Can you work these out from the model? Positions are in its coordinate system, mm. A direction names the side the tool comes from. Coordinates: 2 decimals unless noted, no trailing zeros. Loops run counter-clockwise (first coordinate to the right, second up) from the corner with the lowest first, then second, coordinate; pieces in that order, holes last. Notation, with made-up numbers: (35.5, 18.25) -> (44.5, 18.25) arc R16 ccw to (44.5, 48.25) -> close; hole circle Ø4 at (34, 53). An arc over 180 degrees is marked (long way). Put each result on its own line as item: value. Start each with the question number.
Item 1: If we section it at B-B on y = 0: Please give me the cut outline in (x, z), plus the area to 3 significant figures.
Item 2: For faces 1 (the cylindrical face through (-32.1, -32.14, -5.93)), 2 (the cylindrical face through (41, 41.07, -7.34)), 3 (the flat face through (0, 39.4, -7)), 4 (the cylindrical face through (0.404, -40.972, -10.074)), which set-ups out of +Z, -Z, +X, -X, +Y, -Y let a thin tool reach every point of the face, with its end or its side?
Item 3: If we section it at D-D on y = 24: Please give me the cut outline in (x, z).
Item 4: Will these pins go through, and if not, where does the flat tip stop? P1, Ø6.5, axis at x = -3, y = -28, coming from the +Z side; P2, Ø5.5, axis at y = 0, z = -7, coming from the -X side; P3, Ø1, axis at x = 16, y = 20, coming from the +Z side.
Item 5: We'd pull the mould along Z, two halves only. Please class faces 5 (the flat face through (-39.4, 0, -7)), 6 (the cylindrical face through (0.52, -41.07, -17)), 7 (the flat face through (-18, 33, -6)): pulls with the +Z half, pulls with the -Z half, needs draft (parallel to the pull), parting line crosses it, or undercut.
Item 6: If we section it at A-A on x = 0: Please give me the cut outline in (y, z).
Item 7: Please list where these lines run through material, in increasing order: L1, parallel to Y at x = 16, z = -9; L2, parallel to X at y = -8.5, z = -7; L3, parallel to X at y = 30.5, z = -10. Write a range as from..to.
Item 8: If we section it at C-C on z = -7: State how many separate pieces and enclosed holes the cut face has, plus the area to 3 significant figures.
```python
from build123d import *

# Parameters (mm, degrees)
F0_W      = 85
F0_H      = 85
F0_R      = 2
F3_DEPTH  = 18.5
F4_DEPTH  = 14
F5_R      = 5
F6_R      = 3
F7_R      = 3.1
F8_DEPTH  = 3.1
F9_R      = 3.1
F10_DEPTH = 3.1
F11_R     = 3.1
F12_DEPTH = 3.1
F13_R     = 3.1
F14_DEPTH = 3.1
F15_DEPTH = 1
F18_DEPTH = 48
F19_R     = 1
F20_ANGLE = 180


# Not quite as in the source:
# - a feature names something its author has since deleted; it is built from what else it names


with BuildPart() as f3:
    # F0 (on Top) → F3 (new body)
    with BuildSketch(Plane.XY):
        Rectangle(F0_W, F0_H)
        with BuildLine():
            ThreePointArc((-33, 30), (-32.1213203436, 32.1213203436), (-30, 33))
            Line((-30, 33), (30, 33))
            ThreePointArc((30, 33), (32.1213203436, 32.1213203436), (33, 30))
            Line((33, 30), (33, 24))
            ThreePointArc((33, 24), (32.1213203436, 21.8786796564), (30, 21))
            Line((30, 21), (-30, 21))
            ThreePointArc((-30, 21), (-32.1213203436, 21.8786796564), (-33, 24))
            Line((-33, 24), (-33, 30))
        make_face(mode=Mode.SUBTRACT)
        with Locations((0, 37.75)):
            Circle(F0_R, mode=Mode.SUBTRACT)
        with BuildLine():
            Line((30, 33), (-30, 33))
            ThreePointArc((-30, 33), (-32.1213203436, 32.1213203436), (-33, 30))
            Line((-33, 30), (-33, 24))
            ThreePointArc((-33, 24), (-32.1213203436, 21.8786796564), (-30, 21))
            Line((-30, 21), (30, 21))
            ThreePointArc((30, 21), (32.1213203436, 21.8786796564), (33, 24))
            Line((33, 24), (33, 30))
            ThreePointArc((33, 30), (32.1213203436, 32.1213203436), (30, 33))
        make_face()
        with Locations((0, 37.75)):
            Circle(F0_R)
    extrude(amount=F3_DEPTH)

    # F0 (on Top) → F4 (cut)
    with BuildSketch(Plane.XY):
        with BuildLine():
            Line((30, 33), (-30, 33))
            ThreePointArc((-30, 33), (-32.1213203436, 32.1213203436), (-33, 30))
            Line((-33, 30), (-33, 24))
            ThreePointArc((-33, 24), (-32.1213203436, 21.8786796564), (-30, 21))
            Line((-30, 21), (30, 21))
            ThreePointArc((30, 21), (32.1213203436, 21.8786796564), (33, 24))
            Line((33, 24), (33, 30))
            ThreePointArc((33, 30), (32.1213203436, 32.1213203436), (30, 33))
        make_face()
    extrude(amount=F4_DEPTH, mode=Mode.SUBTRACT)

    # F5
    f5_edges = [f3.edges().sort_by_distance(p)[0] for p in [
        (0, 42.5, 18.5),
        (-42.5, 0, 18.5),
        (0, -42.5, 18.5),
        (42.5, 0, 18.5),
        (42.5, 42.5, 9.25),
        (-42.5, 42.5, 9.25),
        (-42.5, -42.5, 9.25),
        (42.5, -42.5, 9.25),
    ]]
    fillet(f5_edges, radius=F5_R)

    # F6
    f6_edges = [f3.edges().sort_by_distance(p)[0] for p in [
        (0, 33, 14),
        (-32.12132, 32.12132, 14),
        (-33, 27, 14),
        (-32.12132, 21.87868, 14),
        (0, 21, 14),
        (32.12132, 21.87868, 14),
        (33, 27, 14),
        (32.12132, 32.12132, 14),
    ]]
    fillet(f6_edges, radius=F6_R)

    # F7 (on face) → F8 (cut)
    with BuildSketch(Plane.XZ.offset(42.5)):
        with Locations((0, 7)):
            Circle(F7_R)
    extrude(amount=-F8_DEPTH, mode=Mode.SUBTRACT)

    # F9 (on face) → F10 (cut)
    with BuildSketch(Plane(origin=(0, 42.5, 0), x_dir=(-1, 0, 0), z_dir=(0, 1, 0))):
        with Locations((0, 7)):
            Circle(F9_R)
    extrude(amount=-F10_DEPTH, mode=Mode.SUBTRACT)

    # F11 (on face) → F12 (cut)
    with BuildSketch(Plane(origin=(-42.5, 0, 0), x_dir=(0, -1, 0), z_dir=(-1, 0, 0))):
        with Locations((0, 7)):
            Circle(F11_R)
    extrude(amount=-F12_DEPTH, mode=Mode.SUBTRACT)

    # F13 (on face) → F14 (cut)
    with BuildSketch(Plane.YZ.offset(42.5)):
        with Locations((0, 7)):
            Circle(F13_R)
    extrude(amount=-F14_DEPTH, mode=Mode.SUBTRACT)

    # F0 (on Top) → F15 (cut)
    with BuildSketch(Plane.XY):
        with Locations((0, 37.75)):
            Circle(F0_R)
    extrude(amount=F15_DEPTH, mode=Mode.SUBTRACT)

    # F17 (on offset) → F18 (cut)
    with BuildSketch(Plane(origin=(0, 15, 0), x_dir=(-1, 0, 0), z_dir=(0, 1, 0))):
        with BuildLine():
            Line((-33, 0), (-3, 0))
            ThreePointArc((-3, 0), (-18, 13.5), (-33, 0))
        make_face()
        with BuildLine():
            Line((3, 0), (33, 0))
            ThreePointArc((33, 0), (18, 13.5), (3, 0))
        make_face()
    extrude(amount=-F18_DEPTH, mode=Mode.SUBTRACT)

    # F19
    f19_edges = [f3.edges().sort_by_distance(p)[0] for p in [
        (-42.5, 0, 0),
        (-33, -9, 0),
        (-18, 15, 0),
        (-3, -9, 0),
        (-18, -33, 0),
        (3, -9, 0),
        (18, -33, 0),
        (33, -9, 0),
        (18, 15, 0),
        (0, 21, 0),
    ]]
    fillet(f19_edges, radius=F19_R)


with BuildPart() as f3_1:
    # F20: moved
    add(f3.part.rotate(Axis((0, 0, 0), (1, 0, 0)), F20_ANGLE))


solid = f3_1.part
```
Solutions:
1. outline: (-42.5, -13.5) arc R5 ccw to (-37.5, -18.5) -> (37.5, -18.5) arc R5 ccw to (42.5, -13.5) -> (42.5, -10.1) -> (39.4, -10.1) -> (39.4, -3.9) -> (42.5, -3.9) -> (42.5, -1) arc R1 ccw to (41.5, 0) -> (33.87, 0) arc R1 ccw to (32.89, -0.84) arc R15.08 cw to (3.11, -0.84) arc R1 ccw to (2.13, 0) -> (-2.13, 0) arc R1 ccw to (-3.11, -0.84) arc R15.08 cw to (-32.89, -0.84) arc R1 ccw to (-33.87, 0) -> (-41.5, 0) arc R1 ccw to (-42.5, -1) -> (-42.5, -3.9) -> (-39.4, -3.9) -> (-39.4, -10.1) -> (-42.5, -10.1) -> close
1. area: 903 mm^2
2. face 1: +Z
2. face 2: +Z, -Z, +X, +Y
2. face 3: +Y
2. face 4: -Y
3. outline: (-42.5, -13.5) arc R5 ccw to (-37.5, -18.5) -> (37.5, -18.5) arc R5 ccw to (42.5, -13.5) -> (42.5, -1) arc R1 ccw to (41.5, 0) -> (33.87, 0) arc R1 ccw to (32.89, -0.84) arc R15.08 cw to (3.11, -0.84) arc R1 ccw to (2.13, 0) -> (-2.13, 0) arc R1 ccw to (-3.11, -0.84) arc R15.08 cw to (-32.89, -0.84) arc R1 ccw to (-33.87, 0) -> (-41.5, 0) arc R1 ccw to (-42.5, -1) -> close
4. P1: z = -13.73
4. P2: x = -39.4
4. P3: z = -13.29
5. face 5: undercut
5. face 6: pulls with the -Z half
5. face 7: needs draft
6. outline: (-42.5, -13.5) arc R5 ccw to (-37.5, -18.5) -> (37.5, -18.5) arc R5 ccw to (42.5, -13.5) -> (42.5, -10.1) -> (39.4, -10.1) -> (39.4, -3.9) -> (42.5, -3.9) -> (42.5, -1) arc R1 ccw to (41.5, 0) -> (-20, 0) arc R1 ccw to (-21, -1) -> (-21, -11) arc R3 cw to (-24, -14) -> (-30, -14) arc R3 cw to (-33, -11) -> (-33, -1) arc R1 ccw to (-34, 0) -> (-35.75, 0) -> (-35.75, -1) -> (-39.75, -1) -> (-39.75, 0) -> (-41.5, 0) arc R1 ccw to (-42.5, -1) -> (-42.5, -3.9) -> (-39.4, -3.9) -> (-39.4, -10.1) -> (-42.5, -10.1) -> close
7. L1: -42.5..-33, -21..-15, 33..42.5
7. L2: -42.5..-30.4, -5.6..5.6, 30.4..42.5
7. L3: -42.5..-27.66, -8.34..8.34, 27.66..42.5
8. separate pieces: 1
8. enclosed holes: 3
8. area: 3,960 mm^2
